from build123d import *

# Parameters (mm, degrees)
SKETCH_1_W          = 11
SKETCH_1_H          = 5
EXTRUDE_2_DEPTH     = 6
CUT_EXTRUDE_2_DEPTH = 10.552486587
SKETCH_3_R          = 0.6
EXTRUDE_3_DEPTH     = 5.5
SKETCH_4_R          = 0.14862502
EXTRUDE_4_DEPTH     = 4.5


with BuildPart() as part:
    # 草图1 → 拉伸2 (new body)
    with BuildSketch(Plane.XY):
        Rectangle(SKETCH_1_W, SKETCH_1_H)
    extrude(amount=EXTRUDE_2_DEPTH)

    # 草图2 → 切除-拉伸2 (cut, through all)
    with BuildSketch(Plane(origin=(0, 2.5, 0), x_dir=(-1, 0, 0), z_dir=(0, 1, 0))):
        Polygon((-44.7283548, 3), (-7.684787792, 3), (0, 3), (0, -1.817199173), (0, -38.860766181), (-50.624833681, -92.953553513), (-95.353188481, -51.092787332), align=None)
    extrude(amount=-CUT_EXTRUDE_2_DEPTH, mode=Mode.SUBTRACT)

    # 草图3 → 拉伸3 (add)
    with BuildSketch(Plane(origin=(0, 0, 0), x_dir=(0, 0, -1), z_dir=(1, 0, 0))):
        with Locations(Location((-1.3, 0, 0), (0, 0, 270))):
            Circle(SKETCH_3_R)
    extrude(amount=EXTRUDE_3_DEPTH)

    # 草图4 → 拉伸4 (add)
    with BuildSketch(Plane.XY.offset(6)):
        with Locations((-5.13193451, 0.14862502)):
            Circle(SKETCH_4_R)
        with Locations((-2.474169448, 1.757272294)):
            Circle(SKETCH_4_R)
        with Locations((-2.474169448, -1.879669369)):
            Circle(SKETCH_4_R)
    extrude(amount=EXTRUDE_4_DEPTH)


solid = part.part
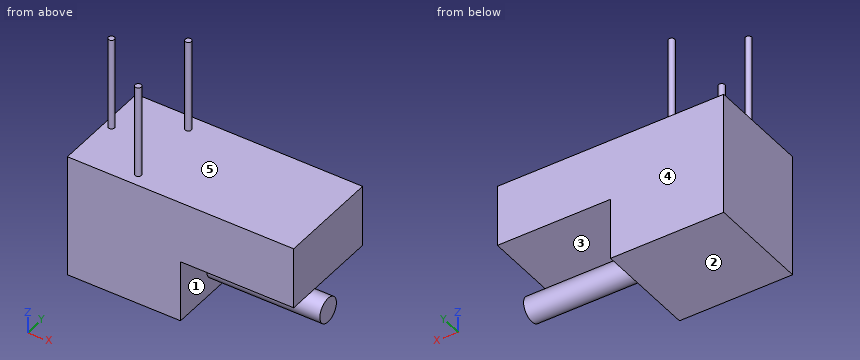
Source: CAD feature listing. Evaluate the final solid. Frame: model axes, mm. Face numbers are marked on the shaded views. A direction names the side the tool comes from. Coordinates: 2 decimals unless noted, no trailing zeros. Write each loop counter-clockwise with the first axis right and the second up, starting at its lowest first coordinate (ties: lowest second). Pieces come first, ordered by that corner, then holes. Notation, with made-up numbers: M -6,81 L -1,81 A13 ccw -1,104 Z; hole C 7.25,78.25 d9. An arc over 180 degrees is marked long. Use a Markdown table: item, result.
1) Section C-C, the plane z = 1.3. Output: boundary loops of the cut face in (x, y), then the cut area to 3 significant figures.
Conclusion:
| item | result |
|---|---|
| outline | M -5.5,-2.5 L 0,-2.5 L 0,-0.6 L 5.5,-0.6 L 5.5,0.6 L 0,0.6 L 0,2.5 L -5.5,2.5 Z |
| area | 34.1 mm^2 |
2) Section B-B, the plane y = 2.1. Output: boundary loops of the cut face in (x, z), then the cut area to 3 significant figures.
Conclusion:
| item | result |
|---|---|
| outline | M -5.5,0 L 0,0 L 0,3 L 5.5,3 L 5.5,6 L -5.5,6 Z |
| area | 49.5 mm^2 |
3) Section D-D, the plane z = 6.5. Output: boundary loops of the cut face in (x, y).
Conclusion:
| item | result |
|---|---|
| outline | C -5.13,0.15 d0.3; C -2.47,-1.88 d0.3; C -2.47,1.76 d0.3 |
4) Section A-A, the plane x = 1.25. Output: boundary loops of the cut face in (y, z), then the cut area to 3 significant figures.
Conclusion:
| item | result |
|---|---|
| outline | M -2.5,3 L 2.5,3 L 2.5,6 L -2.5,6 Z; C 0,1.3 d1.2 |
| area | 16.1 mm^2 |
5) First-contact query: pin 1 Ø1 at (x, z) = (3.5, 8) entering from -Y; pin 2 Ø1.5 at (y, z) = (1.5, 9) entering from +X; pin 3 Ø2.5 at (x, y) = (2.5, 0) entering from +Z. Flat tips, straight axial feed; report the tip coordinate or a pass-through.
Conclusion:
| item | result |
|---|---|
| pin 1 | passes through |
| pin 2 | stops at x = -2.33 |
| pin 3 | stops at z = 6 |
6) Ray query, L1, parallel to Z at x = -0.5, y = -0.7; L2, parallel to Z at x = 1.25, y = -2; L3, parallel to Z at x = 4.25, y = 0.05. Return the intervals inside material, ascending.
Conclusion:
| item | result |
|---|---|
| L1 | z = 0 to 6 |
| L2 | z = 3 to 6 |
| L3 | z = 0.7 to 1.9, 3 to 6 |
7) Reachability of the marked faces 1 and 2 from +Z, -Z, +X, -X, +Y, -Y: full face, straight path, thin tool, end or side. Return the list, or none.
Conclusion:
| item | result |
|---|---|
| face 1 | +X |
| face 2 | -Z, +X, -X, +Y, -Y |
8) Mould query, pull axis Z, two halves, no side actions, for the marked faces 3, 4 and 5. Classes: pulls with the +Z half, pulls with the -Z half, needs draft (parallel to the pull), parting line crosses it, or undercut.
Conclusion:
| item | result |
|---|---|
| face 3 | undercut |
| face 4 | needs draft |
| face 5 | pulls with the +Z half |
